from build123d import *

# Parameters (mm, degrees)
SKETCH1_W           = 44.45
SKETCH1_H           = 12.7
SKETCH1_R           = 1.75
SKETCH1_W_2         = 30.48
BOSS_EXTRUDE1_DEPTH = 3.175
SKETCH2_R           = 1.75
CUT_EXTRUDE1_DEPTH  = 12.192
SKETCH3_W           = 13.97
SKETCH3_H           = 19.05
CUT_EXTRUDE2_DEPTH  = 25.4


with BuildPart() as part:
    # Sketch1 → Boss-Extrude1 (new body)
    # profile 1 of 2: a face of its own
    with BuildSketch(Plane(origin=(0, 0, 0), x_dir=(-1, 0, 0), z_dir=(0, 1, 0))):
        Rectangle(SKETCH1_W, SKETCH1_H)
        with Locations(Location((19.05, 0, 0), (0, 0, 90))):
            Circle(SKETCH1_R, mode=Mode.SUBTRACT)
        with Locations(Location((-19.05, 0, 0), (0, 0, 90))):
            Circle(SKETCH1_R, mode=Mode.SUBTRACT)
    # profile 2 of 2: a face of its own
    with BuildSketch(Plane(origin=(0, 0, 0), x_dir=(-1, 0, 0), z_dir=(0, 1, 0))):
        with Locations((0, 12.7)):
            Rectangle(SKETCH1_W_2, SKETCH1_H)
    extrude(amount=BOSS_EXTRUDE1_DEPTH)

    # Sketch2 → Cut-Extrude1 (cut)
    with BuildSketch(Plane(origin=(0, 3.175, 0), x_dir=(-1, 0, 0), z_dir=(0, 1, 0))):
        with Locations(Location((-11.43, 12.7, 0), (0, 0, 90))):
            Circle(SKETCH2_R)
        with Locations(Location((11.43, 12.7, 0), (0, 0, 90))):
            Circle(SKETCH2_R)
    extrude(amount=-CUT_EXTRUDE1_DEPTH, mode=Mode.SUBTRACT)

    # Sketch3 → Cut-Extrude2 (cut)
    with BuildSketch(Plane(origin=(0, 3.175, 0), x_dir=(-1, 0, 0), z_dir=(0, 1, 0))):
        with Locations((0, 9.525)):
            Rectangle(SKETCH3_W, SKETCH3_H)
    extrude(amount=-CUT_EXTRUDE2_DEPTH, mode=Mode.SUBTRACT)


solid = part.part
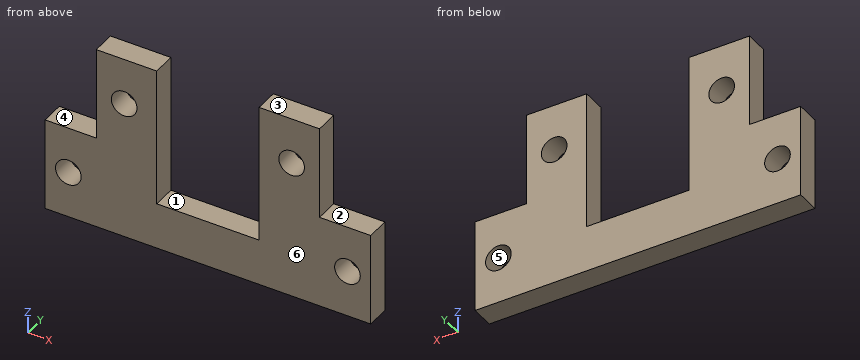
The listing builds one solid part. Answer for the finished solid, in the listing's coordinates (mm). Face numbers are marked on the shaded views. A direction names the side the tool comes from. Round coordinates to 2 decimals unless told otherwise and drop trailing zeros. Loops run counter-clockwise (first coordinate to the right, second up) from the corner with the lowest first, then second, coordinate; pieces in that order, holes last. Notation, with made-up numbers: M -19,10.5 L 28,10.5 A28 cw 28,43.5 Z; hole C 9.5,86.25 d1. An arc over 180 degrees is marked long. Write each question's results on one line, items separated by ' | '. Start each with the question number.
1) Determine the mould class of the marked faces 5 and 6 for opening direction X: pulls with the +X half, pulls with the -X half, needs draft (parallel to the pull), parting line crosses it, or undercut.
2) Find section A-A on x = -19.05. Write down the section's boundary in (y, z) (3 decimals).
3) Find section D-D on z = -0.5. Write down the section's boundary in (x, y) (3 decimals).
4) Find section B-B on z = 15. Write down the section's boundary in (x, y) (3 decimals), plus the area to 3 significant figures.
5) Straight lines are drawn through the part: probe 1 along X at (y, z) = (1.5, 12.7) (3 decimals); probe 2 along X at (y, z) = (1.6, 2) (3 decimals); probe 3 along X at (y, z) = (1.4, 13.5) (3 decimals). For each, find the intervals that lie inside material, in ascending order.
6) Each of these flat-tipped pins is pushed along its axis until it touches: pin 1 (4.5 mm diameter, centred on x = -19.05, z = 0, fed in from -Y); pin 2 (1 mm diameter, centred on x = 2.5, y = 2.5, fed in from +Z); pin 3 (3 mm diameter, centred on x = -11.43, z = 12.7, fed in from +Y); pin 4 (1 mm diameter, centred on x = -20, y = 1.5, fed in from +Z). Where does it stop, or does it pass through?
7) Which of the six approach directions +Z, -Z, +X, -X, +Y, -Y give full straight-line access (tool end or side, diameter ignored) to the marked faces 1, 2, 3 and 4?
8) Find section C-C on y = 2. Write down the section's boundary in (x, z) (3 decimals), plus the area to 3 significant figures.
Final values:
1) face 5: undercut | face 6: needs draft
2) outline: M 0,-6.35 L 3.175,-6.35 L 3.175,-1.75 L 0,-1.75 Z; M 0,1.75 L 3.175,1.75 L 3.175,6.35 L 0,6.35 Z
3) outline: M -22.225,0 L -20.727,0 L -20.727,3.175 L -22.225,3.175 Z; M -17.373,0 L 17.373,0 L 17.373,3.175 L -17.373,3.175 Z; M 20.727,0 L 22.225,0 L 22.225,3.175 L 20.727,3.175 Z
4) outline: M -15.24,0 L -6.985,0 L -6.985,3.175 L -15.24,3.175 Z; M 6.985,0 L 15.24,0 L 15.24,3.175 L 6.985,3.175 Z | area: 52.4 mm²
5) probe 1: -15.24 to -13.18, -9.68 to -6.985, 6.985 to 9.68, 13.18 to 15.24 | probe 2: -22.225 to -6.985, 6.985 to 22.225 | probe 3: -15.24 to -12.986, -9.874 to -6.985, 6.985 to 9.874, 12.986 to 15.24
6) pin 1: y = 0 | pin 2: z = 0 | pin 3: through | pin 4: z = 6.35
7) face 1: +Z, +Y, -Y | face 2: +Z, +X, +Y, -Y | face 3: +Z, +X, -X, +Y, -Y | face 4: +Z, -X, +Y, -Y
8) outline: M -22.225,-6.35 L 22.225,-6.35 L 22.225,6.35 L 15.24,6.35 L 15.24,19.05 L 6.985,19.05 L 6.985,0 L -6.985,0 L -6.985,19.05 L -15.24,19.05 L -15.24,6.35 L -22.225,6.35 Z; hole C -19.05,0 d3.5; hole C -11.43,12.7 d3.5; hole C 11.43,12.7 d3.5; hole C 19.05,0 d3.5 | area: 647 mm²
